from build123d import *

# Parameters (mm, degrees)
ESQUISSE1_W             = 33.5
ESQUISSE1_H             = 25.5
ESQUISSE1_R             = 1.475
ESQUISSE1_W_2           = 27
ESQUISSE1_H_2           = 15
ESQUISSE1_W_3           = 19
ESQUISSE1_W_4           = 8
BOSS_EXTRU_9_DEPTH      = 1
ESQUISSE1_17_W          = 8
ESQUISSE1_17_H          = 15
BOSS_EXTRU_12_DEPTH     = 10
CHANFREIN5_SIZE         = 2
CHANFREIN5_SIZE2        = 3
ESQUISSE6_W             = 3
ESQUISSE6_H             = 4.5
ENL_V_MAT_EXTRU_1_DEPTH = 1
ESQUISSE1_18_W          = 19
ESQUISSE1_18_H          = 15
BOSS_EXTRU_14_DEPTH     = 15


with BuildPart() as part:
    # Esquisse1 → Boss.-Extru.9 (new body)
    # profile 1 of 3: a face of its own
    with BuildSketch(Plane(origin=(0, 0, 0), x_dir=(1, 0, 0), z_dir=(0, 1, 0))):
        with Locations((-5.3869574, 4.310655738)):
            Rectangle(ESQUISSE1_W, ESQUISSE1_H)
        with Locations(Location((8.8630426, 14.560655738, 0), (0, 0, 270))):
            Circle(ESQUISSE1_R, mode=Mode.SUBTRACT)
        with Locations(Location((8.8630426, -5.939344262, 0), (0, 0, 270))):
            Circle(ESQUISSE1_R, mode=Mode.SUBTRACT)
        with Locations(Location((-19.1369574, 14.560655738, 0), (0, 0, 270))):
            Circle(ESQUISSE1_R, mode=Mode.SUBTRACT)
        with Locations(Location((-19.1369574, -5.939344262, 0), (0, 0, 270))):
            Circle(ESQUISSE1_R, mode=Mode.SUBTRACT)
        with Locations((-3.247540984, 3.560655738)):
            Rectangle(ESQUISSE1_W_2, ESQUISSE1_H_2, mode=Mode.SUBTRACT)
    # profile 2 of 3: a face of its own
    with BuildSketch(Plane(origin=(0, 0, 0), x_dir=(1, 0, 0), z_dir=(0, 1, 0))):
        with Locations((-7.247540984, 3.560655738)):
            Rectangle(ESQUISSE1_W_3, ESQUISSE1_H_2)
    # profile 3 of 3: a face of its own
    with BuildSketch(Plane(origin=(0, 0, 0), x_dir=(1, 0, 0), z_dir=(0, 1, 0))):
        with Locations((6.252459016, 3.560655738)):
            Rectangle(ESQUISSE1_W_4, ESQUISSE1_H_2)
    extrude(amount=-BOSS_EXTRU_9_DEPTH)

    # Esquisse1_17 → Boss.-Extru.12 (add)
    with BuildSketch(Plane(origin=(0, 0, 0), x_dir=(1, 0, 0), z_dir=(0, 1, 0))):
        with Locations((6.252459016, 3.560655738)):
            Rectangle(ESQUISSE1_17_W, ESQUISSE1_17_H)
    extrude(amount=BOSS_EXTRU_12_DEPTH)

    # Chanfrein5
    chanfrein5_edges = [part.edges().sort_by_distance(p)[0] for p in [
        (2.252459016, 10, -3.560655738),
        (10.252459016, 10, -3.560655738),
    ]]
    chanfrein5_side = [part.faces().sort_by_distance(p)[0] for p in [
        (6.252459016, 10, -3.560655738),
    ]]
    chamfer(chanfrein5_edges, length=CHANFREIN5_SIZE, length2=CHANFREIN5_SIZE2, reference=chanfrein5_side[0])

    # Esquisse6 → Enl_v. mat.-Extru.1 (cut)
    with BuildSketch(Plane(origin=(10.252459016, 0, 0), x_dir=(0, 0, -1), z_dir=(1, 0, 0))):
        with Locations((3.560655738, 3.25)):
            Rectangle(ESQUISSE6_W, ESQUISSE6_H)
        with Locations((8.560655738, 3.25)):
            Rectangle(ESQUISSE6_W, ESQUISSE6_H)
        with Locations((-1.439344262, 3.25)):
            Rectangle(ESQUISSE6_W, ESQUISSE6_H)
    extrude(amount=-ENL_V_MAT_EXTRU_1_DEPTH, mode=Mode.SUBTRACT)

    # Esquisse1_18 → Boss.-Extru.14 (add)
    with BuildSketch(Plane(origin=(0, 0, 0), x_dir=(1, 0, 0), z_dir=(0, 1, 0))):
        with Locations((-7.247540984, 3.560655738)):
            Rectangle(ESQUISSE1_18_W, ESQUISSE1_18_H)
    extrude(amount=BOSS_EXTRU_14_DEPTH)


solid = part.part
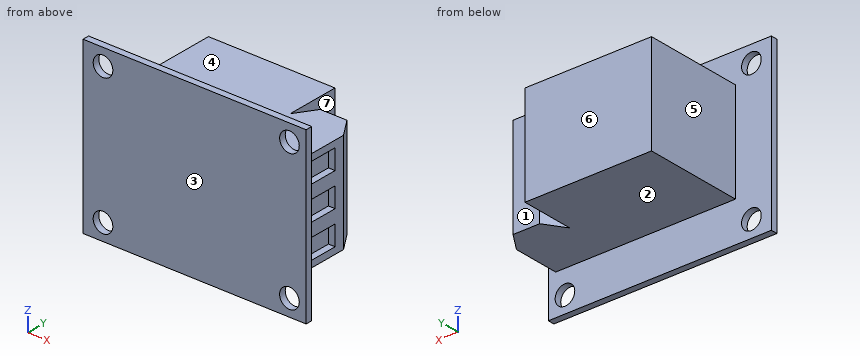
Could you check a few things on this model? Use its own coordinates, in mm. Face numbers are marked on the shaded views. A direction names the side the tool comes from. Round coordinates to 2 decimals unless told otherwise and drop trailing zeros. Write each loop counter-clockwise with the first axis right and the second up, starting at its lowest first coordinate (ties: lowest second). Pieces come first, ordered by that corner, then holes. Notation, with made-up numbers: (58.25, 50) - (95.25, 50) arc R26 cw to (95.25, 82) - close; hole circle Ø6 at (25.5, 15.25). An arc over 180 degrees is marked (long way). Use a Markdown table: item, result.
Q1. Please list where these lines run through material, in increasing order: L1, parallel to Y at x = 0, z = 5.75; L2, parallel to Z at x = -16, y = 5.75; L3, parallel to X at y = 0.5, z = -8.25.
Output values:
| item | result |
|---|---|
| L1 | -1 to 0 |
| L2 | -11.06 to 3.94 |
| L3 | -16.75 to 10.25 |
Q2. I want a section at B-B (y = 3.5). List the corners of the cut face in (x, z) for me, plus the area to 3 significant figures.
Output values:
| item | result |
|---|---|
| outline | (-16.75, -11.06) - (10.25, -11.06) - (10.25, -10.06) - (9.25, -10.06) - (9.25, -7.06) - (10.25, -7.06) - (10.25, -5.06) - (9.25, -5.06) - (9.25, -2.06) - (10.25, -2.06) - (10.25, -0.06) - (9.25, -0.06) - (9.25, 2.94) - (10.25, 2.94) - (10.25, 3.94) - (-16.75, 3.94) - close |
| area | 396 mm2 |
Q3. I want a section at A-A (x = -18.5). List the corners of the cut face in (y, z) for me, plus the area to 3 significant figures.
Output values:
| item | result |
|---|---|
| outline | (-1, -17.06) - (0, -17.06) - (0, -15.89) - (-1, -15.89) - close; (-1, -13.23) - (0, -13.23) - (0, 4.61) - (-1, 4.61) - close; (-1, 7.27) - (0, 7.27) - (0, 8.44) - (-1, 8.44) - close |
| area | 20.2 mm2 |
Q4. For the marked faces 1, 2, 3 and 4, which set-ups out of +Z, -Z, +X, -X, +Y, -Y let a thin tool reach every point of the face, with its end or its side?
Output values:
| item | result |
|---|---|
| face 1 | +Z, -Z, +X, +Y |
| face 2 | -Z, +X, -X, +Y |
| face 3 | +Z, -Z, +X, -X, -Y |
| face 4 | +Z, +X, -X, +Y |
Q5. I want a section at D-D (z = 5.5). List the corners of the cut face in (x, y) for me (3 decimals).
Output values:
| item | result |
|---|---|
| outline | (-22.137, -1) - (-20.545, -1) - (-20.545, 0) - (-22.137, 0) - close; (-17.729, -1) - (7.455, -1) - (7.455, 0) - (-17.729, 0) - close; (10.271, -1) - (11.363, -1) - (11.363, 0) - (10.271, 0) - close |
Q6. Thinking about a two-plate mould opening in X: for the marked faces 5, 6 and 7, which applies, released by +X, released by -X, zero draft, split by the parting line, or undercut?
Output values:
| item | result |
|---|---|
| face 5 | released by -X |
| face 6 | zero draft |
| face 7 | undercut |
Q7. I want a section at C-C (x = 5). List the corners of the cut face in (y, z) for me.
Output values:
| item | result |
|---|---|
| outline | (-1, -17.06) - (0, -17.06) - (0, -11.06) - (10, -11.06) - (10, 3.94) - (0, 3.94) - (0, 8.44) - (-1, 8.44) - close |
Q8. For pin 1 (3.5 mm diameter, centred on x = -19.14, z = 5.94, fed in from +Y); pin 2 (3 mm diameter, centred on y = 4.5, z = 5, fed in from -X); pin 3 (5 mm diameter, centred on x = -18, y = 3, fed in from -Z), each with a flat end and sliding along its axis, tell me the tip position at first contact or that it passes through.
Output values:
| item | result |
|---|---|
| pin 1 | y = 0 |
| pin 2 | x = -16.75 |
| pin 3 | z = -11.06 |
